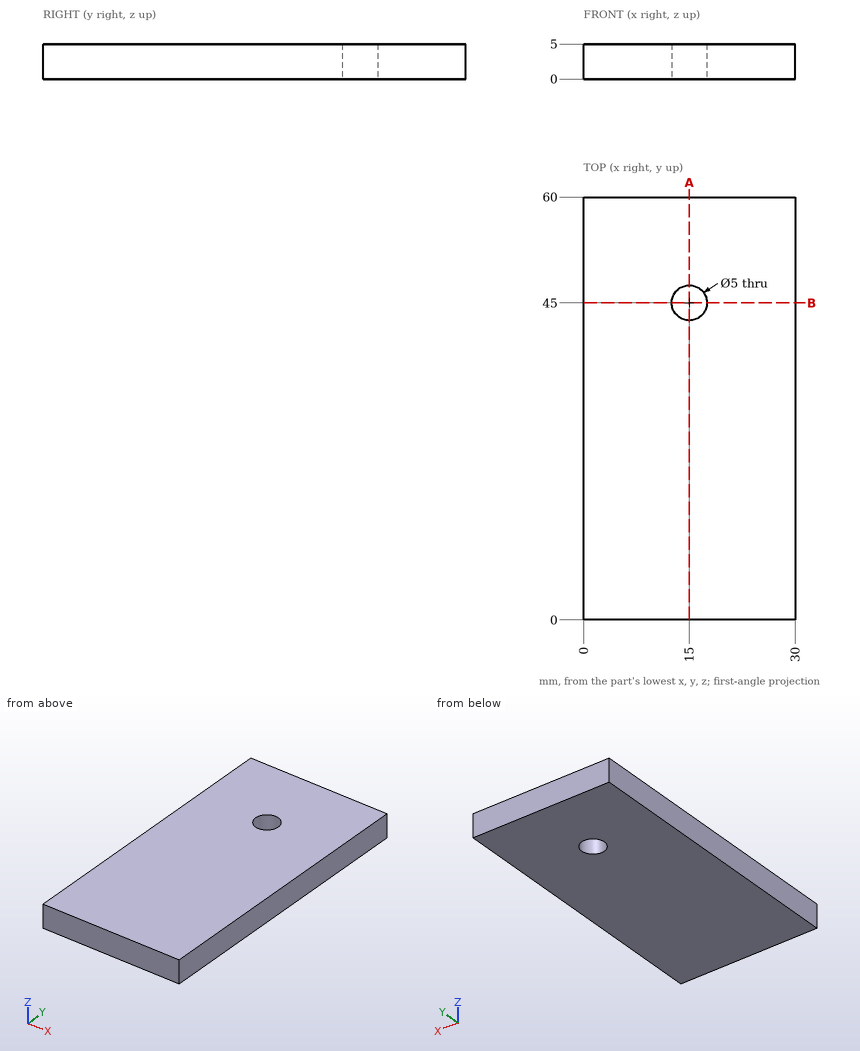
Can you work these out from the drawing? Everything is in mm from the part's minimum corner. Round coordinates to 2 decimals unless told otherwise and drop trailing zeros. Order: outer loops, then holes, each group sorted by start corner. A loop starts at its lowest first (then second) coordinate and runs counter-clockwise, first axis right, second up. Notation, with made-up numbers: M 7.5,49.25 L 55.5,49.25 A19 cw 55.5,76.25 Z; hole C -29.75,58 d9. An arc over 180 degrees is marked long. One line per question, with ' | ' between items.
1) I want a section at A-A, the plane x = 15. Write out the boundary of the cut face in (y, z).
Working result:
outline: M 0,0 L 42.5,0 L 42.5,5 L 0,5 Z; M 47.5,0 L 60,0 L 60,5 L 47.5,5 Z
2) I need wall thicknesses on line 1 along X through (y, z) = (45, 1.35); line 2 along Y through (x, z) = (15, 2.35); line 3 along X through (y, z) = (46.5, 1.55). Which ranges of each line are inside material? Lowest first, please.
Working result:
line 1: 0 to 12.5, 17.5 to 30 | line 2: 0 to 42.5, 47.5 to 60 | line 3: 0 to 13, 17 to 30
3) I want a section at B-B, the plane y = 45. Write out the boundary of the cut face in (x, z).
Working result:
outline: M 0,0 L 12.5,0 L 12.5,5 L 0,5 Z; M 17.5,0 L 30,0 L 30,5 L 17.5,5 Z
4) For pin 1 Ø6.5 at (x, y) = (15, 45) entering from +Z, with a flat end and sliding along its axis, tell me the tip position at first contact or that it passes through.
Working result:
pin 1: z = 5
